Drawing for the job (mm, zero at the part's lowest x, y, z). A direction names the side the tool comes from. Round coordinates to 2 decimals unless told otherwise and drop trailing zeros. Write each loop counter-clockwise with the first axis right and the second up, starting at its lowest first coordinate (ties: lowest second). Pieces come first, ordered by that corner, then holes.
Item 1: Band-saw the part on A-A, the plane y = 19.4. Write the cut outline in (x, z), then the cut area to 3 significant figures.
Item 2: Band-saw the part on B-B, the plane z = 11.5. Write the cut outline in (x, y).
Item 3: 3-axis set-ups, long thin cutter, end or side, ignore diameter. For the marked faces 5, 6, 7 and 8: which of +Z, -Z, +X, -X, +Y, -Y reach the whole face in a straight line?
Item 4: Band-saw the part on D-D, the plane y = 15. Write the cut outline in (x, z) (1 decimal).
Item 5: Drop flat-ended pins along their axis: pin 1 Ø1 at (y, z) = (22.5, 29.5) entering from -X; pin 2 Ø12 at (x, z) = (25.5, 35.5) entering from +Y; pin 3 Ø2 at (x, y) = (8, 11.5) entering from -Z. Give the stop position or say it passes through.
Item 6: Mould opens along Y. For the marked faces 1, 2, 3 and 4 say: +Y half, -Y half, draft (parallel to the pull), parting line (faces both ways), or undercut.
Item 7: Wall check: probe 1 along Y at (x, z) = (19.4, 38.75); probe 2 along Z at (x, y) = (18, 13); probe 3 along Z at (x, y) = (20, 37). Give the ranges that are in metal, low to high.
Item 8: Band-saw the part on C-C, the plane x = 11.5. Write the cut outline in (y, z).
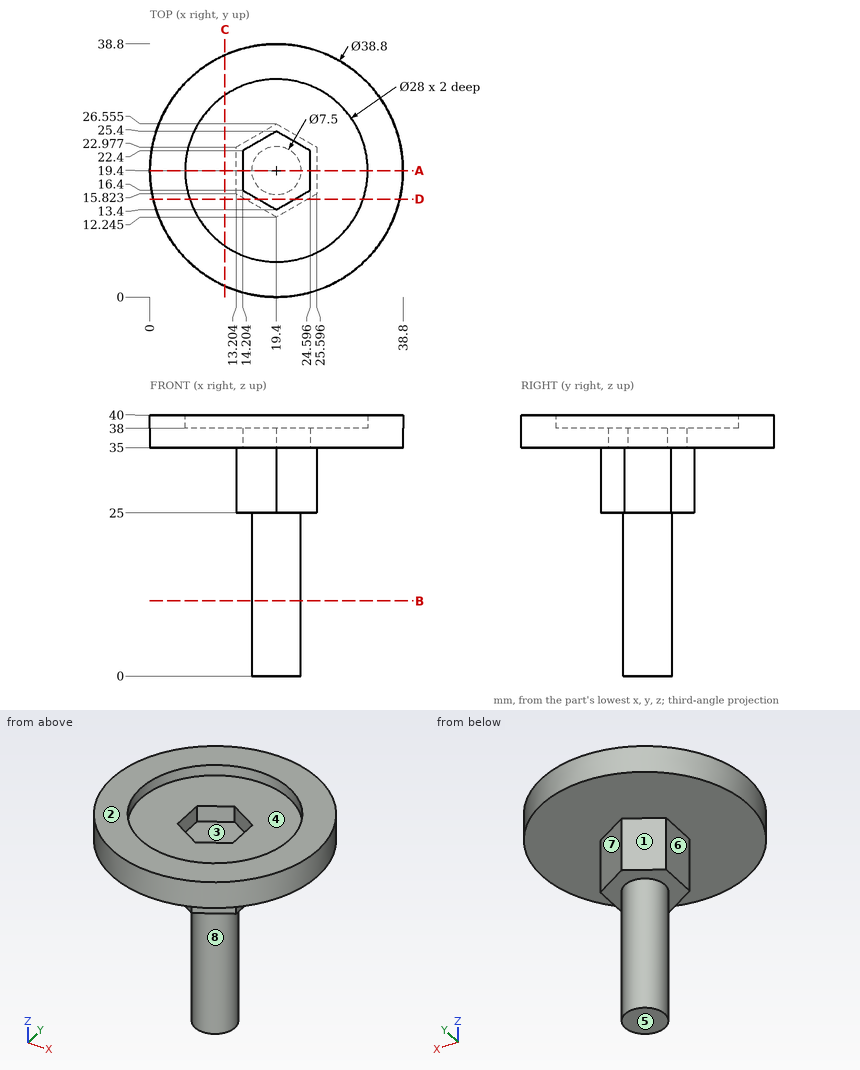
Results:
1. outline: (0, 35) - (13.2, 35) - (13.2, 25) - (15.65, 25) - (15.65, 0) - (23.15, 0) - (23.15, 25) - (25.6, 25) - (25.6, 35) - (38.8, 35) - (38.8, 40) - (33.4, 40) - (33.4, 38) - (24.6, 38) - (24.6, 35) - (14.2, 35) - (14.2, 38) - (5.4, 38) - (5.4, 40) - (0, 40) - close
1. area: 418 mm2
2. outline: circle Ø7.5 at (19.4, 19.4)
3. face 5: -Z, +X, -X, +Y, -Y
3. face 6: -Z, -X, +Y, -Y
3. face 7: -Z, +X, +Y
3. face 8: -Z
4. outline: (0.5, 35) - (14.6, 35) - (14.6, 25) - (24.2, 25) - (24.2, 35) - (38.3, 35) - (38.3, 40) - (32.7, 40) - (32.7, 38) - (22.2, 38) - (22.2, 35) - (16.6, 35) - (16.6, 38) - (6.1, 38) - (6.1, 40) - (0.5, 40) - close
5. pin 1: stops at x = 13.2
5. pin 2: stops at y = 38.8
5. pin 3: stops at z = 35
6. face 1: +Y half
6. face 2: draft
6. face 3: undercut
6. face 4: undercut
7. probe 1: y = 0 to 5.4, 33.4 to 38.8
7. probe 2: z = 35 to 38
7. probe 3: z = 35 to 40
8. outline: (1.68, 35) - (37.12, 35) - (37.12, 40) - (30.96, 40) - (30.96, 38) - (7.84, 38) - (7.84, 40) - (1.68, 40) - close
